Here's the drawing with two shaded views (mm, measured from the low corner). I have some questions. A direction names the side the tool comes from. Give positions to 0.01 mm unless a question says otherwise; leave off trailing zeros. Write each loop counter-clockwise with the first axis right and the second up, starting at its lowest first coordinate (ties: lowest second). Pieces come first, ordered by that corner, then holes. Notation, with made-up numbers: (81, 1.5) - (139, 1.5) arc R25 ccw to (139, 28.5) - close; hole circle Ø4 at (4, 67.5). An arc over 180 degrees is marked (long way). Use one line per item in the form item = value.
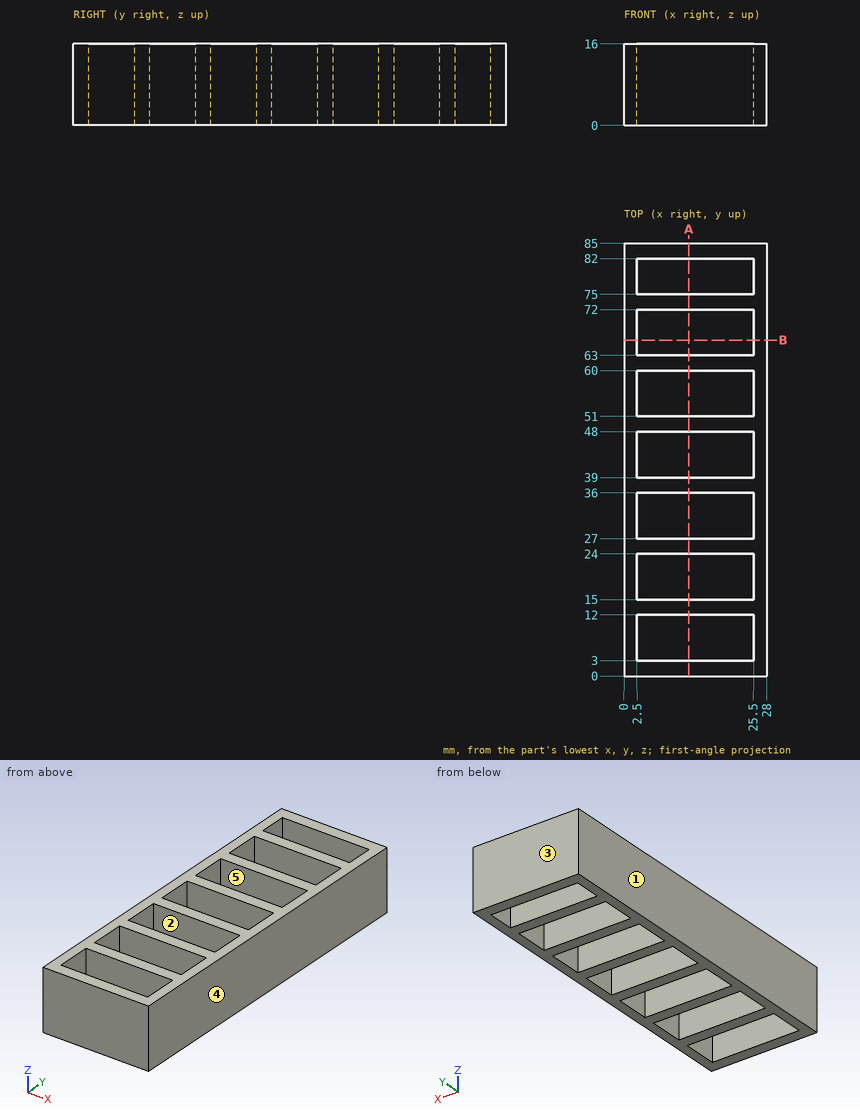
1. Which directions (+Z, -Z, +X, -X, +Y, -Y) give clear straight access to the entire face, cutting with the end or side of a thin tool? Please do the marked faces 1 and 2.
Response values:
face_1 = +Z, -Z, -X, +Y, -Y
face_2 = +Z, -Z
2. Imagine slicing it at B-B, the plane y = 66. List the corners of the cut face in (x, z) for me, and give its area (3 significant figures).
Response values:
outline = (0, 0) - (2.5, 0) - (2.5, 16) - (0, 16) - close; (25.5, 0) - (28, 0) - (28, 16) - (25.5, 16) - close
area = 80.0 mm²
3. If we mould it in two halves opening along X, with no side actions, what happens to the marked faces 3, 4 and 5? For each: pulls with the +X half, pulls with the -X half, needs draft (parallel to the pull), parting line crosses it, or undercut.
Response values:
face_3 = needs draft
face_4 = pulls with the +X half
face_5 = undercut
4. If I drill on line 1 (X direction, y = 71.5, z = 1.5), over which ranges is the centre line in solid material (lowest first)? Write a range as from..to.
Response values:
line_1 = 0..2.5, 25.5..28
5. Imagine slicing it at A-A, the plane x = 12.75. State how many separate pieces and enclosed holes the cut face has, and give its area (3 significant figures).
Response values:
separate_pieces = 8
enclosed_holes = 0
area = 384 mm²
